Could you check a few things on this drawing? It's one solid part, dimensions in mm from its lowest x, y, z. A direction names the side the tool comes from. Coordinates: 2 decimals unless noted, no trailing zeros. Order: outer loops, then holes, each group sorted by start corner. A loop starts at its lowest first (then second) coordinate and runs counter-clockwise, first axis right, second up. Notation, with made-up numbers: (7, -21) -> (50, -21) arc R29 cw to (50, 17) -> close; hole circle Ø11 at (-14, 18). An arc over 180 degrees is marked (long way). Use a Markdown table: item, result. Add a question column.
1. Suppose I cut it at C-C, the plane y = 9. List the corners of the cut face in (x, z) for me, then the cut area to 3 significant figures.
2. Suppose I cut it at A-A, the plane x = 26.35. List the corners of the cut face in (y, z) for me.
3. Suppose I cut it at B-B, the plane z = 2.65. List the corners of the cut face in (x, y) for me.
4. For pin 1 Ø1.2 at (x, z) = (4.5, 2) entering from -Y; pin 2 Ø1.2 at (y, z) = (12.5, 1.5) entering from -X, each with a flat end and sliding along its axis, tell me the tip position at first contact or that it passes through.
5. Suppose I cut it at D-D, the plane y = 12. List the corners of the cut face in (x, z) for me, then the cut area to 3 significant figures.
6. We'd pull the mould along Y, two halves only. Please class the marked faces 1, 2, 3 and 4: pulls with the +Y half, pulls with the -Y half, needs draft (parallel to the pull), parting line crosses it, or undercut.
7. If I drill on line 1 along Y through (x, z) = (16.35, 1.45); line 2 along X through (y, z) = (1, 2.5); line 3 along Y through (x, z) = (2.5, 2.25), over which ranges is the centre line in solid material (lowest first)? Write a range as from..to.
8. For the marked faces 5, 6 and 7, which set-ups out of +Z, -Z, +X, -X, +Y, -Y let a thin tool reach every point of the face, with its end or its side?
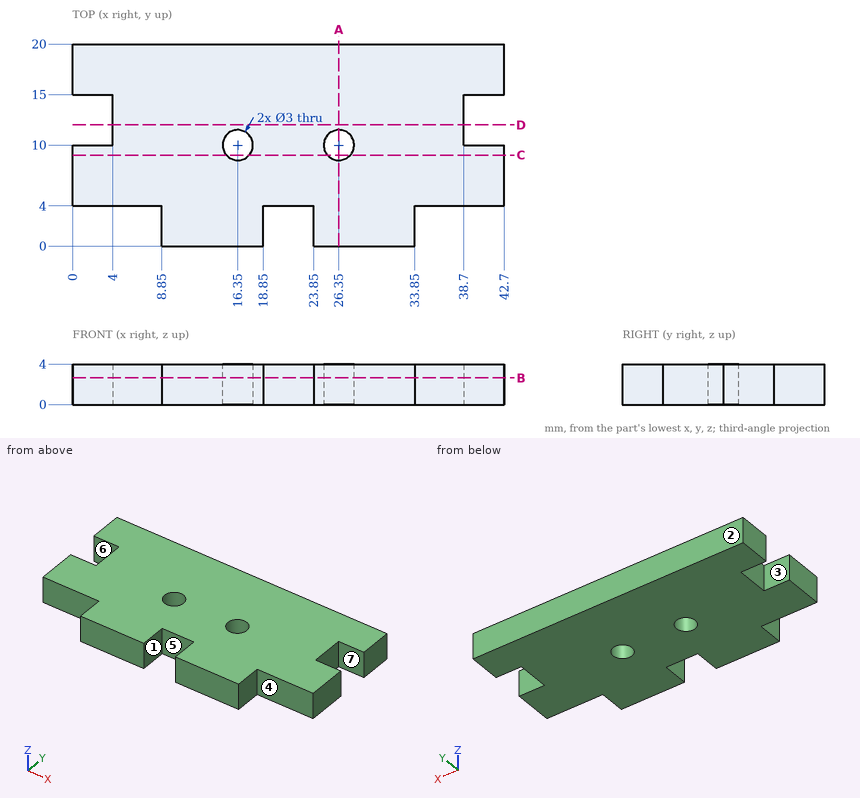
Worked out:
| question | item | result |
|---|---|---|
| 1 | outline | (0, 0) -> (15.23, 0) -> (15.23, 4) -> (0, 4) -> close; (17.47, 0) -> (25.23, 0) -> (25.23, 4) -> (17.47, 4) -> close; (27.47, 0) -> (42.7, 0) -> (42.7, 4) -> (27.47, 4) -> close |
| 1 | area | 153 mm² |
| 2 | outline | (0, 0) -> (8.5, 0) -> (8.5, 4) -> (0, 4) -> close; (11.5, 0) -> (20, 0) -> (20, 4) -> (11.5, 4) -> close |
| 3 | outline | (0, 4) -> (8.85, 4) -> (8.85, 0) -> (18.85, 0) -> (18.85, 4) -> (23.85, 4) -> (23.85, 0) -> (33.85, 0) -> (33.85, 4) -> (42.7, 4) -> (42.7, 10) -> (38.7, 10) -> (38.7, 15) -> (42.7, 15) -> (42.7, 20) -> (0, 20) -> (0, 15) -> (4, 15) -> (4, 10) -> (0, 10) -> close; hole circle Ø3 at (16.35, 10); hole circle Ø3 at (26.35, 10) |
| 4 | pin 1 | stops at y = 4 |
| 4 | pin 2 | stops at x = 4 |
| 5 | outline | (4, 0) -> (38.7, 0) -> (38.7, 4) -> (4, 4) -> close |
| 5 | area | 139 mm² |
| 6 | face 1 | needs draft |
| 6 | face 2 | pulls with the +Y half |
| 6 | face 3 | undercut |
| 6 | face 4 | pulls with the -Y half |
| 7 | line 1 | y = 0..8.5, 11.5..20 |
| 7 | line 2 | x = 8.85..18.85, 23.85..33.85 |
| 7 | line 3 | y = 4..10, 15..20 |
| 8 | face 5 | +Z, -Z, -Y |
| 8 | face 6 | +Z, -Z, -X |
| 8 | face 7 | +Z, -Z, +X |
